Can you work these out from the model? Positions are in its coordinate system, mm. Face numbers are marked on the shaded views. Coordinates: 2 decimals unless noted, no trailing zeros. Answer in a Markdown table with one row per item. Add a question column.
1. Will these pins go through, and if not, where does the flat tip stop? pin 1 (12 mm diameter, centred on x = 18.5, z = 11.5, fed in from -Y); pin 2 (5 mm diameter, centred on x = -28.5, z = 6.5, fed in from -Y); pin 3 (10 mm diameter, centred on x = 5, z = 27, fed in from +Y).
2. Imagine slicing it at B-B on x = 0. State how many separate pieces and enclosed holes the cut face has, plus the area to 3 significant figures.
3. If I drill on line 1 along Z through (x, y) = (0, 30.75); line 2 along Y through (x, z) = (0, 10); line 3 along Y through (x, z) = (-17.5, 4), over which ranges is the centre line in solid material (lowest first)? Write a range as [from, to].
4. We'd pull the mould along X, two halves only. Please class the marked faces 1, 2 and 3: pulls with the +X half, pulls with the -X half, needs draft (parallel to the pull), parting line crosses it, or undercut.
from build123d import *

# Parameters (mm, degrees)
F0_R          = 44.45
F0_R_2        = 26.9875
F1_DEPTH      = 31.75
F2_R          = 3.175
F3_DEPTH      = 44.451
F3_DEPTH_BACK = 44.451
F4_R          = 1.27
F5_SIZE       = 3.175


with BuildPart() as f1:
    # F0 (on Top) → F1 (new body)
    with BuildSketch(Plane.XY):
        Circle(F0_R)
        Circle(F0_R_2, mode=Mode.SUBTRACT)
    extrude(amount=F1_DEPTH)

    # F2 (on Front) → F3 (cut, two sides)
    with BuildSketch(Plane.XZ) as f3_sk:
        with Locations((0, 15.875)):
            Circle(F2_R)
    extrude(amount=-F3_DEPTH, mode=Mode.SUBTRACT)
    extrude(f3_sk.sketch, amount=F3_DEPTH_BACK, mode=Mode.SUBTRACT)

    # F4
    f4_edges = [f1.edges().sort_by_distance(p)[0] for p in [
        (-44.45, 0, 31.75),
        (-44.45, 0, 0),
    ]]
    fillet(f4_edges, radius=F4_R)

    # F5
    f5_edges = [f1.edges().sort_by_distance(p)[0] for p in [
        (-26.9875, 0, 31.75),
        (-26.9875, 0, 0),
    ]]
    chamfer(f5_edges, length=F5_SIZE)


solid = f1.part
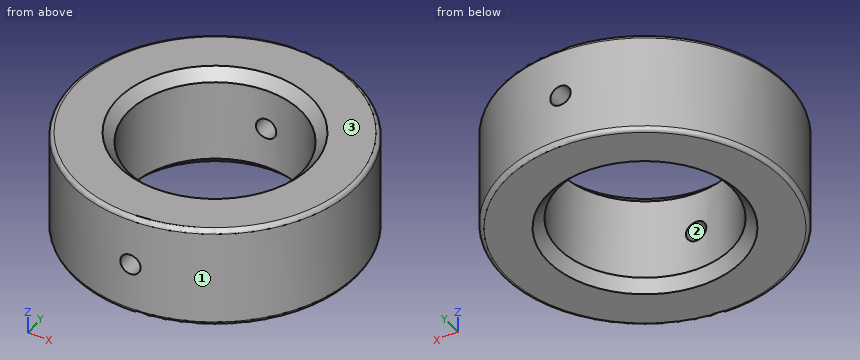
Answers follow:
| question | item | result |
|---|---|---|
| 1 | pin 1 | stops at y = -42.66 |
| 1 | pin 2 | stops at y = -36.05 |
| 1 | pin 3 | stops at y = 44.45 |
| 2 | separate pieces | 4 |
| 2 | enclosed holes | 0 |
| 2 | area | 866 mm² |
| 3 | line 1 | z = [0, 12.7], [19.05, 31.75] |
| 3 | line 2 | y = [-44.45, -26.99], [26.99, 44.45] |
| 3 | line 3 | y = [-40.86, -20.54], [20.54, 40.86] |
| 4 | face 1 | parting line crosses it |
| 4 | face 2 | undercut |
| 4 | face 3 | needs draft |
